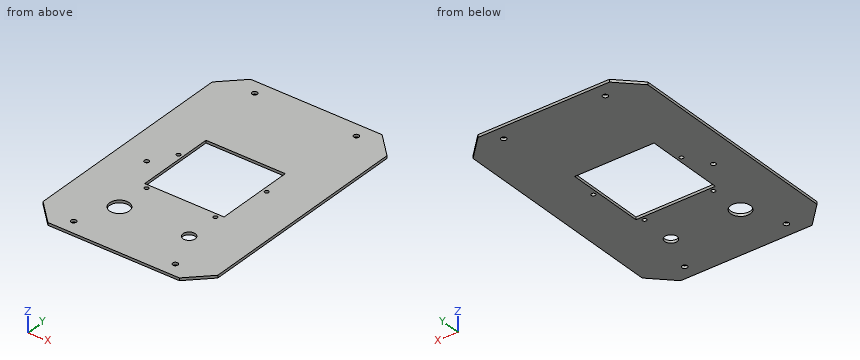
```python
from build123d import *

# Parameters (mm, degrees)
BASE_DEPTH              = 3
ESQUISSE2_R             = 3
ENL_V_MAT_EXTRU_1_DEPTH = 4
ENL_V_MAT_EXTRU_2_REACH = 5
ESQUISSE3_R             = 11.25
ESQUISSE3_R_2           = 7
ENL_V_MAT_EXTRU_3_REACH = 5
ESQUISSE4_R             = 2.625
ENL_V_MAT_EXTRU_4_REACH = 5
ESQUISSE5_W             = 90.5
ESQUISSE5_H             = 90.5
ESQUISSE6_R             = 2.25
ENL_V_MAT_EXTRU_5_DEPTH = 10


with BuildPart() as part:
    # Esquisse1 → Base (new body)
    with BuildSketch(Plane.XY):
        Polygon((24.748737342, 24.748737342), (0, 0), (-150, 0), (-174.748737342, 24.748737342), (-174.748737342, 274.748737342), (-150, 299.497474683), (0, 299.497474683), (24.748737342, 274.748737342), align=None)
    extrude(amount=BASE_DEPTH)

    # Esquisse2 → Enlèv. mat.-Extru.1 (cut, through all)
    with BuildSketch(Plane(origin=(0, 0, 0), x_dir=(-1, 0, 0), z_dir=(0, 0, -1))):
        with Locations((132.998737342, 283.497474683)):
            Circle(ESQUISSE2_R)
        with Locations((132.998737342, 16)):
            Circle(ESQUISSE2_R)
        with Locations((17.001262658, 16)):
            Circle(ESQUISSE2_R)
        with Locations((17.001262658, 283.497474683)):
            Circle(ESQUISSE2_R)
    extrude(amount=-ENL_V_MAT_EXTRU_1_DEPTH, mode=Mode.SUBTRACT)

    # Esquisse3 → Enlèv. mat.-Extru.2 (cut, up to next)
    with BuildSketch(Plane(origin=(0, 0, 0), x_dir=(-1, 0, 0), z_dir=(0, 0, -1)), mode=Mode.PRIVATE) as enl_v_mat_extru_2_sk1:
        with Locations((114.748737342, 60)):
            Circle(ESQUISSE3_R)
    enl_v_mat_extru_2_tool1 = extrude(enl_v_mat_extru_2_sk1.sketch, amount=-ENL_V_MAT_EXTRU_2_REACH, mode=Mode.PRIVATE) & part.part
    add(enl_v_mat_extru_2_tool1.solids().sort_by_distance((-114.748737, 60, 0))[0], mode=Mode.SUBTRACT)
    # Esquisse3 → Enlèv. mat.-Extru.2 (cut, up to next)
    with BuildSketch(Plane(origin=(0, 0, 0), x_dir=(-1, 0, 0), z_dir=(0, 0, -1)), mode=Mode.PRIVATE) as enl_v_mat_extru_2_sk2:
        with Locations((35.251262658, 60)):
            Circle(ESQUISSE3_R_2)
    enl_v_mat_extru_2_tool2 = extrude(enl_v_mat_extru_2_sk2.sketch, amount=-ENL_V_MAT_EXTRU_2_REACH, mode=Mode.PRIVATE) & part.part
    add(enl_v_mat_extru_2_tool2.solids().sort_by_distance((-35.251263, 60, 0))[0], mode=Mode.SUBTRACT)

    # Esquisse4 → Enlèv. mat.-Extru.3 (cut, up to next)
    with BuildSketch(Plane(origin=(0, 0, 0), x_dir=(-1, 0, 0), z_dir=(0, 0, -1)), mode=Mode.PRIVATE) as enl_v_mat_extru_3_sk1:
        with Locations((141.498737342, 134.75)):
            Circle(ESQUISSE4_R)
    enl_v_mat_extru_3_tool1 = extrude(enl_v_mat_extru_3_sk1.sketch, amount=-ENL_V_MAT_EXTRU_3_REACH, mode=Mode.PRIVATE) & part.part
    add(enl_v_mat_extru_3_tool1.solids().sort_by_distance((-141.498737, 134.75, 0))[0], mode=Mode.SUBTRACT)

    # Esquisse5 → Enlèv. mat.-Extru.4 (cut, up to next)
    with BuildSketch(Plane.XY.offset(3), mode=Mode.PRIVATE) as enl_v_mat_extru_4_sk1:
        with Locations((-75, 149.748737342)):
            Rectangle(ESQUISSE5_W, ESQUISSE5_H)
    enl_v_mat_extru_4_tool1 = extrude(enl_v_mat_extru_4_sk1.sketch, amount=-ENL_V_MAT_EXTRU_4_REACH, mode=Mode.PRIVATE) & part.part
    add(enl_v_mat_extru_4_tool1.solids().sort_by_distance((-75, 149.748737, 3))[0], mode=Mode.SUBTRACT)

    # Esquisse6 → Enlèv. mat.-Extru.5 (cut)
    with BuildSketch(Plane(origin=(0, 0, 0), x_dir=(-1, 0, 0), z_dir=(0, 0, -1))):
        with Locations((125.25, 160.998737342)):
            Circle(ESQUISSE6_R)
        with Locations((35.75, 99.498737342)):
            Circle(ESQUISSE6_R)
        with Locations((114.25, 99.498737342)):
            Circle(ESQUISSE6_R)
        with Locations((24.75, 160.998737342)):
            Circle(ESQUISSE6_R)
    extrude(amount=-ENL_V_MAT_EXTRU_5_DEPTH, mode=Mode.SUBTRACT)


solid = part.part
```
Could you check a few things on this model? Use its own coordinates, in mm. Round coordinates to 2 decimals unless told otherwise and drop trailing zeros. Order: outer loops, then holes, each group sorted by start corner. A loop starts at its lowest first (then second) coordinate and runs counter-clockwise, first axis right, second up. Notation, with made-up numbers: (-5, 30.5) -> (12, 30.5) arc R16 cw to (12, 55.5) -> close; hole circle Ø10 at (73.25, -40). An arc over 180 degrees is marked (long way). One line per question, with ' | ' between items.
Q1. If we section it at C-C on z = 0.6: Give the number of separate pieces and of enclosed holes in the cut face, plus the area to 3 significant figures.
Computed values:
separate pieces: 1 | enclosed holes: 12 | area: 49,600 mm²
Q2. If I drill on line 1 (Y direction, x = -78, z = 2.45); line 2 (X direction, y = 113, z = 1.75); line 3 (Y direction, x = -24.75, z = 1.4), over which ranges is the centre line in solid material (lowest first)? Write a range as from..to.
Computed values:
line 1: 0..104.5, 195..299.5 | line 2: -174.75..-120.25, -29.75..24.75 | line 3: 0..158.75, 163.25..299.5
Q3. If we section it at A-A on y = 60: Write out the boundary of the cut face in (x, z), plus the area to 3 significant figures.
Computed values:
outline: (-174.75, 0) -> (-126, 0) -> (-126, 3) -> (-174.75, 3) -> close; (-103.5, 0) -> (-42.25, 0) -> (-42.25, 3) -> (-103.5, 3) -> close; (-28.25, 0) -> (24.75, 0) -> (24.75, 3) -> (-28.25, 3) -> close | area: 489 mm²
Q4. If we section it at B-B on x = -85: Write out the boundary of the cut face in (y, z), plus the area to 3 significant figures.
Computed values:
outline: (0, 0) -> (104.5, 0) -> (104.5, 3) -> (0, 3) -> close; (195, 0) -> (299.5, 0) -> (299.5, 3) -> (195, 3) -> close | area: 627 mm²
